Geometry: final body of the model. Coordinates: model frame, mm. A direction names the side the tool comes from. Round coordinates to 2 decimals unless told otherwise and drop trailing zeros. Write each loop counter-clockwise with the first axis right and the second up, starting at its lowest first coordinate (ties: lowest second). Pieces come first, ordered by that corner, then holes. Notation, with made-up numbers: (-25.5, 21.25) -> (-5.5, 21.25) arc R19 ccw to (-5.5, 32.25) -> close; hole circle Ø5 at (-14, 76). An arc over 180 degrees is marked (long way). Use one line per item in the form item = value. Start each with the question number.
1. Line query: L1, parallel to X at y = -10, z = 11.25; L2, parallel to Z at x = -15, y = -3.75; L3, parallel to Y at x = -14, z = 18.75. Output: solid intervals per line, ascending.
2. Reachability of faces 4 (the face through (-4.268, 2, 24)), 5 (the face through (-16.018, -7, 12)), 6 (the face through (-4.268, -7, 2)), 7 (the face through (-24.268, 5, 9)), 8 (the face through (-21, -12.564, 7)) from +Z, -Z, +X, -X, +Y, -Y: full face, straight path, thin tool, end or side. Return the list, or none.
3. Cut plane B-B, the plane x = -26.5. Return the cut outline in (y, z).
4. Cut plane D-D, the plane z = 14.5. Return the cut outline in (x, y), plus the area to 3 significant figures.
5. Draft query along Y for faces 1 (the face through (-20, -2, 19)), 2 (the face through (-30, -0.564, 9)), 3 (the face through (-25.822, -8.296, 9.367)). Return one class per face: pulls with the +Y half, pulls with the -Y half, needs draft (parallel to the pull), parting line crosses it, or undercut.
6. Pin query (flat end, axial travel): pin 1 Ø8 at (x, y) = (-25, 2) entering from +Z; pin 2 Ø5 at (x, z) = (0.5, 6.5) entering from -Y; pin 3 Ø8 at (y, z) = (-8.5, 11.5) entering from +X. Return the tip coordinate at first contact, or that it passes through.
7. Cut plane C-C, the plane y = 5.5. Return the cut outline in (x, z).
8. Cut plane A-A, the plane y = -3.75. Return the cut outline in (x, z).
Autodesk Inventor part; units mm, degrees
ref_plane "YZ Plane" through (0, 0, 0) normal (1, 0, 0) x (0, 1, 0)
ref_plane "XZ Plane" through (0, 0, 0) normal (0, 1, 0) x (-1, 0, 0)
ref_plane "XY Plane" through (0, 0, 0) normal (0, 0, 1) x (1, 0, 0)
sketch "草图1" plane through (0, 0, 0) normal (0, 0, 1) x (1, 0, 0)
  line L0 (-22.2679, -12.5636) -> (3.7321, -12.5636)
  line L1 (-24.2679, 7.4364) -> (5.7321, 7.4364)
  line L2 (5.7321, 7.4364) -> (5.7321, -12.5636)
  line L3 (5.7321, -12.5636) -> (-24.2679, -12.5636)
  line L4 (-24.2679, -12.5636) -> (-24.2679, 7.4364)
  point P0 (-22.2679, -12.5636)
  point P1 (3.7321, -12.5636)
  dimension "d4" = 30
  dimension "d5" = 20
extrude "拉伸1" add sketch "草图1" along normal blind 19
sketch "草图2" plane through (0, 0, 0) normal (0, 0, -1) x (-1, 0, 0)
  line L0 (24.2679, 7.4364) -> (24.2679, -12.5636)
  line L1 (24.2679, -12.5636) -> (31.2679, -12.5636)
  line L2 (31.2679, -12.5636) -> (31.2679, -0.5636)
  line L3 (31.2679, -0.5636) -> (24.2679, -0.5636)
  line L4 (24.2679, -0.5636) -> (24.2679, -12.5636)
  point P0 (0, 0)
  dimension "d6" = 7
  dimension "d7" = 12
extrude "拉伸2" add sketch "草图2" against normal up to surface (19 mm away)
sketch "草图3" plane through (0, 0, 0) normal (0, 0, -1) x (-1, 0, 0)
  circle A0 centre (-0.6256, 1.5535) radius 3
  circle A1 centre (26.4728, -5.3671) radius 3
  point P0 (0, 0)
  dimension "d10" = 6
  dimension "d11" = 6
extrude "拉伸3" cut sketch "草图3" against normal blind 40
sketch "草图4" plane through (5.7321, -12.5636, 0) normal (1, 0, 0) x (0, 0, -1)
  line L0 (-19, 0) -> (-4, 0)
  line L1 (-4, 0) -> (-4, 10)
  line L2 (-4, 10) -> (-19, 10)
  line L3 (-19, 10) -> (-19, 0)
  point P0 (0, 12.5636)
  dimension "d14" = 10
  dimension "d15" = 15
extrude "拉伸4" cut sketch "草图4" against normal blind 21.75
chamfer "倒角1" distance 4 angle 45 1 edges at (-24.2679, -0.5636, 9.5)
sketch "草图5" plane through (5.7321, -12.5636, 0) normal (1, 0, 0) x (0, 0, -1)
  line L0 (-4, 0) -> (-19, 0)
  line L1 (-4, 0) -> (0, 0)
  line L2 (0, 0) -> (0, 10)
  line L3 (0, 10) -> (-4, 10)
  line L4 (-4, 10) -> (-4, 0)
  line L5 (0, 0) -> (0, 20)
  line L6 (-19, 10) -> (-4, 10)
  point P0 (0, 12.5636)
extrude "拉伸5" cut sketch "草图5" against normal blind 10
sketch "草图6" plane through (5.7321, -2.5636, 0) normal (0, -1, 0) x (1, 0, 0)
  line L0 (0, 0) -> (0, 19)
  line L1 (0, 0) -> (-8, 0)
  line L2 (-8, 0) -> (-8, 25.7509)
  line L3 (-8, 25.7509) -> (0, 25.7509)
  line L4 (0, 25.7509) -> (0, 0)
  line L5 (-12.3, 25.7509) -> (0, 25.7509)
  line L6 (-21.75, 19) -> (0, 19)
  line L7 (-8, 25.7509) -> (-10, 25.7509)
  line L8 (-10, 25.7509) -> (-10, 19)
  line L9 (-10, 19) -> (-8, 19)
  line L10 (-8, 19) -> (-8, 25.7509)
  point P0 (-5.7321, 0)
  point P1 (-8, 19)
  dimension "d23" = 8
  dimension "d28" = 10
extrude "拉伸6" add sketch "草图6" against normal up to surface (10 mm away)
sketch "草图8" plane through (0, 0, 0) normal (0, 0, -1) x (-1, 0, 0)
  circle A0 centre (-0.6256, 1.5535) radius 3
  point P0 (0, 0)
extrude "拉伸7" cut sketch "草图8" against normal blind 42.75
fillet "圆角1" radius 4 1 edges at (-4.2679, 2.4364, 19)
properties part number "固定传动"
Outcome:
q1.L1 = -31.27 to -16.02
q1.L2 = 0 to 4
q1.L3 = -2.56 to 7.44
q2.face_4 = +Z, -X, +Y, -Y
q2.face_5 = +Z, +X, -Y
q2.face_6 = +Z, -Z, +X, -Y
q2.face_7 = +Z, -Z, -X, +Y
q2.face_8 = +Z, -Z, +X, -X, -Y
q3.outline = (-12.56, 0) -> (-8.37, 0) -> (-8.37, 19) -> (-12.56, 19) -> close; (-2.37, 0) -> (1.2, 0) -> (1.2, 19) -> (-2.37, 19) -> close
q4.outline = (-31.27, -12.56) -> (-16.02, -12.56) -> (-16.02, -2.56) -> (5.73, -2.56) -> (5.73, 7.44) -> (-24.27, 7.44) -> (-24.27, 3.44) -> (-28.27, -0.56) -> (-31.27, -0.56) -> close; hole circle Ø6 at (-26.47, -5.37); hole circle Ø6 at (0.63, 1.55)
q4.area = 418 mm^2
q5.face_1 = needs draft
q5.face_2 = pulls with the +Y half
q5.face_3 = undercut
q6.pin_1 = 19
q6.pin_2 = -2.56
q6.pin_3 = -16.02
q7.outline = (-24.27, 0) -> (5.73, 0) -> (5.73, 25.75) -> (-4.27, 25.75) -> (-4.27, 23) arc R4 cw to (-8.27, 19) -> (-24.27, 19) -> close
q8.outline = (-31.27, 0) -> (-29, 0) -> (-29, 19) -> (-31.27, 19) -> close; (-23.95, 0) -> (-4.27, 0) -> (-4.27, 4) -> (-16.02, 4) -> (-16.02, 19) -> (-23.95, 19) -> close
